Geometry check sheet. Reference: the model listing, model coordinates, mm. Round coordinates to 2 decimals unless told otherwise and drop trailing zeros. Write each loop counter-clockwise with the first axis right and the second up, starting at its lowest first coordinate (ties: lowest second). Pieces come first, ordered by that corner, then holes. Notation, with made-up numbers: (81, 69) -> (104, 69) arc R25 ccw to (104, 108) -> close; hole circle Ø7 at (38.5, 77.5). An arc over 180 degrees is marked (long way). Return JSON: item names as keys, results as strings. Group by question number.
from build123d import *

# Parameters (mm, degrees)
BOSS_EXTRUDE1_DEPTH = 9.525
SKETCH3_R           = 2.032
CUT_EXTRUDE1_DEPTH  = 2.7
SKETCH4_R           = 1.000000032
CUT_EXTRUDE2_DEPTH  = 49.829451626
FILLET2_SIZE        = 6


with BuildPart() as part:
    # Sketch1 → Boss-Extrude1 (new body)
    with BuildSketch(Plane(origin=(0, 0, 0), x_dir=(1, 0, 0), z_dir=(0, 1, 0))):
        Polygon((-29.626544256, -8.559809399), (-45.282501527, -6.441378612), (-42.600711235, 13.378005859), (-26.876432388, 11.317015404), align=None)
    extrude(amount=BOSS_EXTRUDE1_DEPTH)

    # Sketch3 → Cut-Extrude1 (cut)
    with BuildSketch(Plane(origin=(1.004349985, 0, -7.662664899), x_dir=(-0.9915193653276276, 0, -0.12995902500518686), z_dir=(0.12995902500518686, 0, -0.9915193653276276))):
        with Locations((40.946022732, 5.969)):
            Circle(SKETCH3_R)
    extrude(amount=-CUT_EXTRUDE1_DEPTH, mode=Mode.SUBTRACT)

    # Sketch4 → Cut-Extrude2 (cut, through all)
    with BuildSketch(Plane(origin=(0.653460617, 0, -4.985562613), x_dir=(-0.9915193653276276, 0, -0.12995902500518688), z_dir=(0.12995902500518688, 0, -0.9915193653276276))):
        with Locations((40.946022732, 5.969)):
            Circle(SKETCH4_R)
    extrude(amount=-CUT_EXTRUDE2_DEPTH, mode=Mode.SUBTRACT)

    # Fillet2
    # a fillet whose section is not a circle: 6 mm, written as the material it takes off along each edge
    with BuildSketch(Plane(origin=(-47.293844247, 9.525, 21.305916966), x_dir=(0.9909692235697757, 0, 0.13408951464419594), z_dir=(0.13408951464419594, 0, -0.9909692235697757))) as fillet2_piece_1:
        with BuildLine():
            add(Edge.make_bspline([(FILLET2_SIZE, 0), (FILLET2_SIZE * 0.831801948466, 0), (FILLET2_SIZE * 0.663603896932, 0), (FILLET2_SIZE * 0.292893218813, FILLET2_SIZE * 0.0716919198361), (FILLET2_SIZE * 0.0716919198361, FILLET2_SIZE * 0.292893218813), (0, FILLET2_SIZE * 0.663603896932), (0, FILLET2_SIZE * 0.831801948466), (0, FILLET2_SIZE)], knots=[0, 0, 0, 0, 0, 0, 0.5, 0.5, 1, 1, 1, 1, 1, 1], degree=5))
            Line((0, FILLET2_SIZE), (0, 0))
            Line((0, 0), (FILLET2_SIZE, 0))
        make_face()
    extrude(amount=50, mode=Mode.SUBTRACT)
    with BuildSketch(Plane(origin=(-47.293844247, 0, 21.305916966), x_dir=(0.9909692235697757, 0, 0.13408951464419594), z_dir=(0.13408951464419594, 0, -0.9909692235697757))) as fillet2_piece_2:
        with BuildLine():
            add(Edge.make_bspline([(FILLET2_SIZE, 0), (FILLET2_SIZE * 0.831801948466, 0), (FILLET2_SIZE * 0.663603896932, 0), (FILLET2_SIZE * 0.292893218813, -FILLET2_SIZE * 0.0716919198361), (FILLET2_SIZE * 0.0716919198361, -FILLET2_SIZE * 0.292893218813), (0, -FILLET2_SIZE * 0.663603896932), (0, -FILLET2_SIZE * 0.831801948466), (0, -FILLET2_SIZE)], knots=[0, 0, 0, 0, 0, 0, 0.5, 0.5, 1, 1, 1, 1, 1, 1], degree=5))
            Line((0, -FILLET2_SIZE), (0, 0))
            Line((0, 0), (FILLET2_SIZE, 0))
        make_face()
    extrude(amount=50, mode=Mode.SUBTRACT)


solid = part.part
1) Sectioned sample at B-B on x = -31.5. Enter the section's corners in (y, z) (3 decimals), and give its area (3 significant figures).
2) Mould release check, pull along X, two halves, no side actions. Record for faces 1 (the face through (-40.81, 5.09, -10.42)), 2 (the face through (-37.331, 4.696, 7.517)), 3 (the face through (-33, 9.525, -2)): +X half, -X half, draft (parallel to the pull), parting line (faces both ways), or undercut.
3) Sectioned sample at A-A on x = -28.75. Enter the section's corners in (y, z) (3 decimals).
4) Material ranges on probe 1 along X at (y, z) = (5.5, -9); probe 2 along Y at (x, z) = (-40.75, -6.5); probe 3 along Y at (x, z) = (-38.5, -1.25), recorded low to high. Write a range as [from, to].
5) Go/stop test with flat-tipped pins: P1, Ø1, axis at x = -32.5, y = 4.5, coming from the +Z side; P2, Ø3, axis at y = 4.5, z = -8, coming from the +X side; P3, Ø2, axis at x = -31.5, y = 1, coming from the +Z side. Record where each tip stops, or that it passes through.
Evaluation:
{
 "1": {"outline": "(0, -11.923) -> (9.525, -11.923) -> (9.525, 8.306) -> (0, 8.306) -> close", "area": "193 mm2"},
 "2": {"face 1": "undercut", "face 2": "-X half", "face 3": "draft"},
 "3": {"outline": "(0, -11.563) -> (9.525, -11.563) -> (9.525, 2.224) -> (0, 2.224) -> close"},
 "4": {"probe 1": "x = [-43.09, -41.01], [-39.23, -27.2]", "probe 2": "y = [0.42, 5.02], [6.92, 9.1]", "probe 3": "y = [0, 9.52]"},
 "5": {"P1": "stops at z = 8.24", "P2": "stops at x = -27.13", "P3": "stops at z = 8.44"}
}
